```python
from build123d import *

# Parameters (mm, degrees)
SKETCH1_W                = 47.752
SKETCH1_H                = 25.4
SKETCH1_R                = 1.27
BOSS_EXTRUDE1_DEPTH      = 2.286
BOSS_EXTRUDE2_DEPTH      = 0.508
BOSS_EXTRUDE2_DEPTH_BACK = 5.08
CUT_EXTRUDE1_DEPTH       = 4.064


with BuildPart() as part:
    # Sketch1 → Boss-Extrude1 (new body)
    with BuildSketch(Plane(origin=(0, 0, 0), x_dir=(1, 0, 0), z_dir=(0, 1, 0))):
        Rectangle(SKETCH1_W, SKETCH1_H)
        with Locations(Location((-21.59, 10.033, 0), (0, 0, 270))):
            Circle(SKETCH1_R, mode=Mode.SUBTRACT)
        with Locations(Location((21.59, 10.033, 0), (0, 0, 270))):
            Circle(SKETCH1_R, mode=Mode.SUBTRACT)
        with Locations(Location((-21.59, -10.033, 0), (0, 0, 270))):
            Circle(SKETCH1_R, mode=Mode.SUBTRACT)
        with Locations(Location((21.59, -10.033, 0), (0, 0, 270))):
            Circle(SKETCH1_R, mode=Mode.SUBTRACT)
    extrude(amount=BOSS_EXTRUDE1_DEPTH)

    # Sketch2 → Boss-Extrude2 (add, two sides: drawn at the far end of the back side and taken through both)
    with BuildSketch(Plane(origin=(23.876, 0, 0), x_dir=(0, 0, -1), z_dir=(1, 0, 0)).offset(-BOSS_EXTRUDE2_DEPTH_BACK)):
        with BuildLine():
            Line((-3.556, 5.08), (3.556, 5.08))
            ThreePointArc((3.556, 5.08), (4.953, 3.683), (3.556, 2.286))
            Line((3.556, 2.286), (-3.556, 2.286))
            ThreePointArc((-3.556, 2.286), (-4.953, 3.683), (-3.556, 5.08))
        make_face()
    extrude(amount=BOSS_EXTRUDE2_DEPTH + BOSS_EXTRUDE2_DEPTH_BACK)

    # Sketch3 → Cut-Extrude1 (cut)
    with BuildSketch(Plane(origin=(24.384, 0, 0), x_dir=(0, 0, -1), z_dir=(1, 0, 0))):
        with BuildLine():
            Line((-3.556, 4.318), (3.556, 4.318))
            ThreePointArc((3.556, 4.318), (4.191, 3.683), (3.556, 3.048))
            Line((3.556, 3.048), (-3.556, 3.048))
            ThreePointArc((-3.556, 3.048), (-4.191, 3.683), (-3.556, 4.318))
        make_face()
    extrude(amount=-CUT_EXTRUDE1_DEPTH, mode=Mode.SUBTRACT)


solid = part.part
```
Geometry check sheet. Reference: the model listing, model coordinates, mm. A direction names the side the tool comes from. Give positions to 0.01 mm unless a question says otherwise; leave off trailing zeros. Order: outer loops, then holes, each group sorted by start corner. A loop starts at its lowest first (then second) coordinate and runs counter-clockwise, first axis right, second up. Notation, with made-up numbers: (32, 52) -> (77, 52) arc R15 cw to (77, 68) -> close; hole circle Ø4 at (-36, 16.5). An arc over 180 degrees is marked (long way). Write each question's results on one line, items separated by ' | '. Start each with the question number.
(1) Gauge pin test, flat ends, axial feed: P1, Ø1.2, axis at x = 22.5, z = 0.5, coming from the -Y side; P2, Ø1.5, axis at x = -21.59, z = -10.033, coming from the +Y side; P3, Ø1.8, axis at y = 1, z = 0.5, coming from the +X side; P4, Ø12.5, axis at x = -3, z = 2.5, coming from the +Y side. Record the tip position at first contact, or that the pin passes through.
(2) Mould release check, pull along Y, two halves, no side actions. Record for faces 1 (the face through (23.876, 1, 0)), 2 (the face through (22.38, 3.67, 4.19)), 3 (the face through (0, 0, 0)): pulls with the +Y half, pulls with the -Y half, needs draft (parallel to the pull), parting line crosses it, or undercut.
(3) Sectioned sample at B-B (x = 21.59). Enter the section's corners in (y, z) (3 decimals).
(4) Scan lines: line 1 (X direction, y = 1.3, z = 9.5); line 2 (Y direction, x = 9, z = -6); line 3 (X direction, y = 1.7, z = 1.75). Record each from-to range of solid material in increasing order.
(5) Sectioned sample at A-A (x = -21.59). Enter the section's corners in (y, z), plus the area to 3 significant figures.
(6) Sectioned sample at D-D (z = -10). Enter the section's corners in (x, y), plus the area to 3 significant figures.
(7) Sectioned sample at C-C (y = 0.5). Enter the section's corners in (x, z).
(8) Access from +Z, -Z, +X, -X, +Y, -Y to the whole of each face (thin tool, end or side, straight path). Record for faces 4 (the face through (0, 1, -12.7)), 5 (the face through (18.796, 4, 0)), 6 (the face through (22.38, 3.7, -4.19)).
Answer below:
1) P1: y = 0 | P2: through | P3: x = 23.88 | P4: y = 2.29
2) face 1: needs draft | face 2: undercut | face 3: pulls with the -Y half
3) outline: (0, -12.7) -> (2.286, -12.7) -> (2.286, -11.303) -> (0, -11.303) -> close; (0, -8.763) -> (2.286, -8.763) -> (2.286, -3.556) arc R1.397 ccw to (5.08, -3.556) -> (5.08, 3.556) arc R1.397 ccw to (2.286, 3.556) -> (2.286, 8.763) -> (0, 8.763) -> close; (0, 11.303) -> (2.286, 11.303) -> (2.286, 12.7) -> (0, 12.7) -> close; hole (3.048, -3.556) arc R0.635 ccw to (4.318, -3.556) -> (4.318, 3.556) arc R0.635 ccw to (3.048, 3.556) -> close
4) line 1: -23.88 to -22.74, -20.44 to 20.44, 22.74 to 23.88 | line 2: 0 to 2.29 | line 3: -23.88 to 23.88
5) outline: (0, -12.7) -> (2.29, -12.7) -> (2.29, -11.3) -> (0, -11.3) -> close; (0, -8.76) -> (2.29, -8.76) -> (2.29, 8.76) -> (0, 8.76) -> close; (0, 11.3) -> (2.29, 11.3) -> (2.29, 12.7) -> (0, 12.7) -> close | area: 46.5 mm2
6) outline: (-23.88, 0) -> (-22.86, 0) -> (-22.86, 2.29) -> (-23.88, 2.29) -> close; (-20.32, 0) -> (20.32, 0) -> (20.32, 2.29) -> (-20.32, 2.29) -> close; (22.86, 0) -> (23.88, 0) -> (23.88, 2.29) -> (22.86, 2.29) -> close | area: 97.6 mm2
7) outline: (-23.88, -12.7) -> (23.88, -12.7) -> (23.88, 12.7) -> (-23.88, 12.7) -> close; hole circle Ø2.54 at (-21.59, -10.03); hole circle Ø2.54 at (-21.59, 10.03); hole circle Ø2.54 at (21.59, -10.03); hole circle Ø2.54 at (21.59, 10.03)
8) face 4: -Z, +X, -X, +Y, -Y | face 5: +Z, -Z, -X, +Y | face 6: +X
